```python
from build123d import *

# Parameters (mm, degrees)
F0_W     = 25.35
F0_H     = 31.05
F0_R     = 1.5
F1_DEPTH = 5
F3_DEPTH = 11.05
F5_DEPTH = 14


with BuildPart() as f1:
    # F0 (on Top) → F1 (new body)
    with BuildSketch(Plane.XY):
        with Locations((-2.675, 4.475)):
            Rectangle(F0_W, F0_H)
        with Locations((6.35, -1.8)):
            Circle(F0_R, mode=Mode.SUBTRACT)
    extrude(amount=F1_DEPTH)

    # F2 (on face) → F3 (join)
    with BuildSketch(Plane.XY.offset(5)):
        Polygon((-10.35, 20), (-15.35, 20), (-15.35, -11.05), (10, -11.05), (10, -7.05), (-10.35, -7.05), align=None)
    extrude(amount=F3_DEPTH)

    # F4 (on face) → F5 (join)
    with BuildSketch(Plane.YZ.offset(10)):
        Polygon((-7.05, 16.05), (-11.05, 16.05), (-11.05, 0), (20, 0), (20, 5), (-7.05, 5), align=None)
    extrude(amount=F5_DEPTH)


solid = f1.part
```
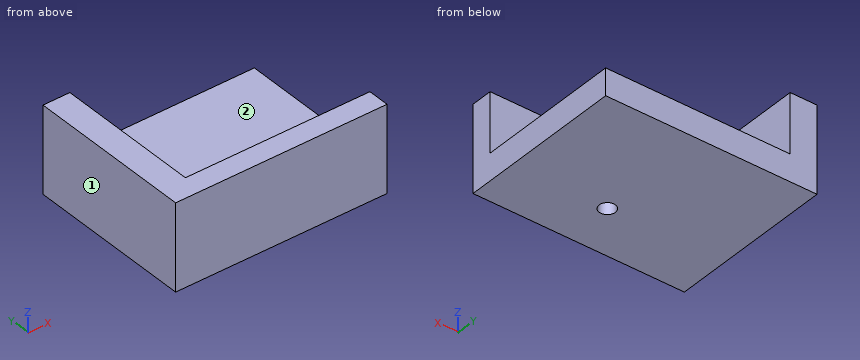
Check sheet for the modelled part. Datum: model origin and axes. Units: mm. Face numbers are marked on the shaded views. A direction names the side the tool comes from. Coordinates: 2 decimals unless noted, no trailing zeros. Loops run counter-clockwise (first coordinate to the right, second up) from the corner with the lowest first, then second, coordinate; pieces in that order, holes last.
1) Sectioned sample at B-B (y = -1.8). Record the boundary of the cut face in (x, z).
2) Sectioned sample at A-A (x = 6.35). Record the boundary of the cut face in (y, z).
3) Sectioned sample at C-C (z = 13.75). Record the boundary of the cut face in (x, y), and give its area (3 significant figures).
4) Material ranges on probe 1 along Y at (x, z) = (6.35, 3.35); probe 2 along X at (y, z) = (16, 15.75); probe 3 along Z at (x, y) = (11.5, 9), recorded low to high.
5) Gauge pin test, flat ends, axial feed: pin 1 (12 mm diameter, centred on x = 12, y = 16.5, fed in from +Z); pin 2 (3 mm diameter, centred on x = 5, z = 12.5, fed in from +Y); pin 3 (9 mm diameter, centred on y = 5, z = 11.5, fed in from +X). Record the tip position at first contact, or that the pin passes through.
6) Access from +Z, -Z, +X, -X, +Y, -Y to the whole of each face (thin tool, end or side, straight path). Record for the marked faces 1 and 2.
Check sheet entries:
1. outline: (-15.35, 0) - (4.85, 0) - (4.85, 5) - (-10.35, 5) - (-10.35, 16.05) - (-15.35, 16.05) - close; (7.85, 0) - (24, 0) - (24, 5) - (7.85, 5) - close
2. outline: (-11.05, 0) - (-3.3, 0) - (-3.3, 5) - (-7.05, 5) - (-7.05, 16.05) - (-11.05, 16.05) - close; (-0.3, 0) - (20, 0) - (20, 5) - (-0.3, 5) - close
3. outline: (-15.35, -11.05) - (24, -11.05) - (24, -7.05) - (-10.35, -7.05) - (-10.35, 20) - (-15.35, 20) - close
3. area: 293 mm2
4. probe 1: y = -11.05 to -3.3, -0.3 to 20
4. probe 2: x = -15.35 to -10.35
4. probe 3: z = 0 to 5
5. pin 1: stops at z = 5
5. pin 2: stops at y = -7.05
5. pin 3: stops at x = -10.35
6. face 1: +Z, -Z, -X, +Y, -Y
6. face 2: +Z, +X, +Y
